Build history of the part. All positions in model axes, mm. A direction names the side the tool comes from. Round coordinates to 2 decimals unless told otherwise and drop trailing zeros. Write each loop counter-clockwise with the first axis right and the second up, starting at its lowest first coordinate (ties: lowest second). Pieces come first, ordered by that corner, then holes. Notation, with made-up numbers: (21, 52) -> (56, 52) arc R12 ccw to (56, 57) -> close; hole circle Ø7 at (1, 43). An arc over 180 degrees is marked (long way). Answer in a Markdown table with one row per item.
```python
from build123d import *

# Parameters (mm, degrees)
BOSS_EXTRUDE1_DEPTH  = 19
SKETCH6_R            = 2
CUT_EXTRUDE2_DEPTH   = 16
SKETCH10_W           = 8
SKETCH10_H           = 1
BOSS_EXTRUDE14_DEPTH = 1
BOSS_EXTRUDE15_DEPTH = 2
SKETCH13_R           = 3
CUT_EXTRUDE3_DEPTH   = 5


with BuildPart() as part:
    # Sketch1 → Boss-Extrude1 (new body)
    with BuildSketch(Plane.XY):
        Polygon((19, 0), (-19, 0), (-19, 13), (-27, 13), (-27, 15), (-19, 15), (-19, 35), (19, 35), (19, 15), (27, 15), (27, 13), (19, 13), align=None)
    extrude(amount=BOSS_EXTRUDE1_DEPTH)

    # Sketch6 → Cut-Extrude2 (cut, through all)
    with BuildSketch(Plane(origin=(0, 15, 0), x_dir=(1, 0, 0), z_dir=(0, 1, 0))):
        with Locations((25.2, -15)):
            Circle(SKETCH6_R)
        with Locations((25.2, -4)):
            Circle(SKETCH6_R)
        with Locations((-25.2, -4)):
            Circle(SKETCH6_R)
        with Locations((-25.2, -15)):
            Circle(SKETCH6_R)
    extrude(amount=-CUT_EXTRUDE2_DEPTH, mode=Mode.SUBTRACT)

    # Sketch10 → Boss-Extrude14 (add)
    with BuildSketch(Plane.XZ.offset(-13)):
        with Locations((-23, 9.5)):
            Rectangle(SKETCH10_W, SKETCH10_H)
        with Locations((23, 9.5)):
            Rectangle(SKETCH10_W, SKETCH10_H)
    extrude(amount=BOSS_EXTRUDE14_DEPTH)

    # Sketch12 → Boss-Extrude15 (add)
    with BuildSketch(Plane.XZ):
        with BuildLine():
            Line((-14, 18.5), (6, 18.5))
            ThreePointArc((6, 18.5), (18.486832981, 9.5), (6, 0.5))
            Line((6, 0.5), (-14, 0.5))
            Line((-14, 0.5), (-14, 18.5))
        make_face()
    extrude(amount=BOSS_EXTRUDE15_DEPTH)

    # Sketch13 → Cut-Extrude3 (cut)
    with BuildSketch(Plane.XZ.offset(2)):
        with Locations((9, 9.5)):
            Circle(SKETCH13_R)
    extrude(amount=-CUT_EXTRUDE3_DEPTH, mode=Mode.SUBTRACT)


solid = part.part
```
Q1. Saw through at C-C on x = -22.5. Write the cut outline in (y, z), plus the area to 3 significant figures.
A:
| item | result |
|---|---|
| outline | (12, 9) -> (13, 9) -> (13, 0) -> (15, 0) -> (15, 19) -> (13, 19) -> (13, 10) -> (12, 10) -> close |
| area | 39.0 mm² |
Q2. Wall check: line 1 (Z direction, x = -25.2, y = 13.5); line 2 (X direction, y = 13.9, z = 4); line 3 (X direction, y = 8.5, z = 15.25). Give the ranges that are in metal, low to high. Write a range as [from, to].
A:
| item | result |
|---|---|
| line 1 | [0, 2], [6, 13], [17, 19] |
| line 2 | [-23.2, 23.2] |
| line 3 | [-19, 19] |
Q3. Drop flat-ended pins along their axis: P1, Ø2, axis at y = 19, z = 10.5, coming from the -X side; P2, Ø2.5, axis at x = -21, z = 15.5, coming from the -Y side; P3, Ø12, axis at x = -19.5, y = 5.5, coming from the +Z side; P4, Ø1.1, axis at x = 23, z = 9.5, coming from the -Y side. Give the stop position or say it passes through.
A:
| item | result |
|---|---|
| P1 | x = -19 |
| P2 | y = 13 |
| P3 | z = 19 |
| P4 | y = 12 |
Q4. Two-plate mould, pull along X, no slides. Class faces 4 (the flat face through (9, 3, 10)), 5 (the flat face through (-1.3, 0, 0.3)), 6 (the cylindrical face through (-23.2, 14.01, 4.08)), 7 (the flat face through (-27, 14, 9)): released by +X, released by -X, zero draft, split by the parting line, or undercut.
A:
| item | result |
|---|---|
| face 4 | undercut |
| face 5 | zero draft |
| face 6 | undercut |
| face 7 | released by -X |
Q5. Saw through at B-B on z = 15. Write the cut outline in (x, y).
A:
| item | result |
|---|---|
| outline | (-23.2, 13) -> (-19, 13) -> (-19, 0) -> (-14, 0) -> (-14, -2) -> (16.73, -2) -> (16.73, 0) -> (19, 0) -> (19, 13) -> (23.2, 13) -> (23.2, 15) -> (19, 15) -> (19, 35) -> (-19, 35) -> (-19, 15) -> (-23.2, 15) -> close |
Q6. Which spindle directions (+Z, -Z, +X, -X, +Y, -Y) get a long thin tool onto all of the face, cutting with end or side? Do faces 1 (the flat face through (-22, 13, 4)), 2 (the cylindrical face through (11.77, 0.46, 8.35)), 3 (the flat face through (-19, 25, 9)). Say none if no direction does.
A:
| item | result |
|---|---|
| face 1 | -Z, -X, -Y |
| face 2 | -Y |
| face 3 | +Z, -Z, -X, +Y |
Q7. Saw through at A-A on x = 25.2. Write the cut outline in (y, z).
A:
| item | result |
|---|---|
| outline | (12, 9) -> (13, 9) -> (13, 6) -> (15, 6) -> (15, 13) -> (13, 13) -> (13, 10) -> (12, 10) -> close; (13, 0) -> (15, 0) -> (15, 2) -> (13, 2) -> close; (13, 17) -> (15, 17) -> (15, 19) -> (13, 19) -> close |
Q8. Saw through at D-D on y = 30. Write the cut outline in (x, z), plus the area to 3 significant figures.
A:
| item | result |
|---|---|
| outline | (-19, 0) -> (19, 0) -> (19, 19) -> (-19, 19) -> close |
| area | 722 mm² |
